Can you work these out from the model? Positions are in its coordinate system, mm. A direction names the side the tool comes from. Coordinates: 2 decimals unless noted, no trailing zeros. Order: outer loops, then holes, each group sorted by start corner. A loop starts at its lowest first (then second) coordinate and runs counter-clockwise, first axis right, second up. Notation, with made-up numbers: (21.25, -39) -> (32.25, -39) arc R30 cw to (32.25, -11) -> close; hole circle Ø5 at (-35, -14). An arc over 180 degrees is marked (long way). Answer as a JSON object with one key per item and string values. Group by question number.
(1) I want a section at D-D, the plane z = 10.5. List the corners of the cut face in (x, y) for me.
(2) Which directions (+Z, -Z, +X, -X, +Y, -Y) give clear straight access to the entire face, cutting with the end or side of a thin tool? Please do faces 4 (the flat face through (-6, 41, 150)), 5 (the cylindrical face through (-38.663, 1.702, 81.438)).
(3) I need wall thicknesses on line 1 (Y direction, x = 0, z = 50); line 2 (Y direction, x = 9, z = 43); line 3 (X direction, y = 2.5, z = 89.5). Which ranges of each line are inside material? Lowest first, please.
(4) I want a section at C-C, the plane z = 33.5. List the corners of the cut face in (x, y) for me, plus the area to 3 significant figures.
(5) I want a section at A-A, the plane x = 0. List the corners of the cut face in (y, z) for me, plus the area to 3 significant figures.
(6) If we mould it in two halves opening along Y, with no side actions, what happens to faces 1 (the cylindrical face through (20.765, -39.923, 76.266)), 2 (the flat face through (0, 0, 6.5)), 3 (the flat face through (-1, 1, 0))? For each: pulls with the +Y half, pulls with the -Y half, needs draft (parallel to the pull), parting line crosses it, or undercut.
(7) For pin 1 (4 mm diameter, centred on x = 22, y = 11, fed in from +Z); pin 2 (12 mm diameter, centred on y = -12.5, z = 34, fed in from -X); pin 3 (6 mm diameter, centred on x = -14, y = 2.5, fed in from -Z); pin 4 (1 mm diameter, centred on x = -2, z = 37, fed in from -Y) (3 decimals), each with a flat end and sliding along its axis, tell me the tip position at first contact or that it passes through.
from build123d import *

# Parameters (mm, degrees)
F0_R     = 45
F1_DEPTH = 150
F2_R     = 38.7
F4_DEPTH = 143.5
F5_R     = 2.5
F6_R     = 7


with BuildPart() as f1:
    # F0 (on Top) → F1 (new body)
    with BuildSketch(Plane.XY):
        Circle(F0_R)
    extrude(amount=F1_DEPTH)

    # F2 (on face) → F4 (cut, through all)
    with BuildSketch(Plane.XY.offset(150)):
        Circle(F2_R)
    extrude(amount=-F4_DEPTH, mode=Mode.SUBTRACT)

    # F5
    f5_edges = [f1.edges().sort_by_distance(p)[0] for p in [
        (-45, 0, 150),
        (-38.7, 0, 150),
    ]]
    fillet(f5_edges, radius=F5_R)

    # F6
    f6_edges = [f1.edges().sort_by_distance(p)[0] for p in [
        (-38.7, 0, 6.5),
        (-45, 0, 0),
    ]]
    fillet(f6_edges, radius=F6_R)


solid = f1.part
Computed values:
{
 "1": {"outline": "circle Ø90 at (0, 0); hole circle Ø76.05 at (0, 0)"},
 "2": {"face 4": "+Z, +X, -X, +Y, -Y", "face 5": "+Z"},
 "3": {"line 1": "y = -45 to -38.7, 38.7 to 45", "line 2": "y = -44.09 to -37.64, 37.64 to 44.09", "line 3": "x = -44.93 to -38.62, 38.62 to 44.93"},
 "4": {"outline": "circle Ø90 at (0, 0); hole circle Ø77.4 at (0, 0)", "area": "1,660 mm2"},
 "5": {"outline": "(-45, 7) arc R7 ccw to (-38, 0) -> (38, 0) arc R7 ccw to (45, 7) -> (45, 147.5) arc R2.5 ccw to (42.5, 150) -> (41.2, 150) arc R2.5 ccw to (38.7, 147.5) -> (38.7, 13.5) arc R7 cw to (31.7, 6.5) -> (-31.7, 6.5) arc R7 cw to (-38.7, 13.5) -> (-38.7, 147.5) arc R2.5 ccw to (-41.2, 150) -> (-42.5, 150) arc R2.5 ccw to (-45, 147.5) -> close", "area": "2,390 mm2"},
 "6": {"face 1": "parting line crosses it", "face 2": "undercut", "face 3": "needs draft"},
 "7": {"pin 1": "stops at z = 6.5", "pin 2": "stops at x = -44.53", "pin 3": "stops at z = 0", "pin 4": "stops at y = -44.975"}
}
